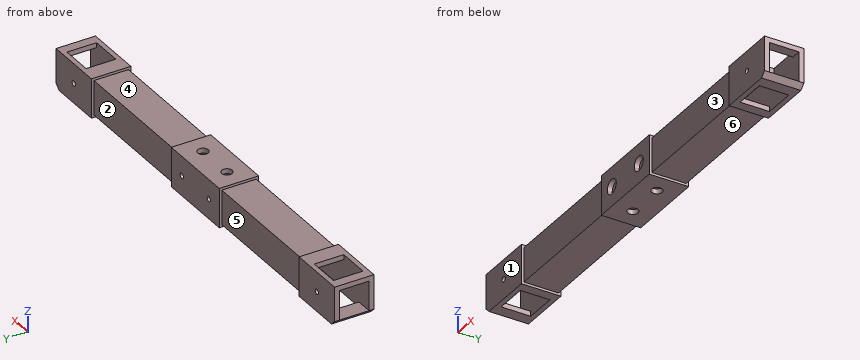
```python
from build123d import *

# Parameters (mm, degrees)
SKETCH1_W               = 50.8
SKETCH1_H               = 50.8
SKETCH1_W_2             = 38.1
SKETCH1_H_2             = 38.1
EXTRUDE1_DEPTH          = 355.6
F_1_2_CLEARANCE_HOLE1_D = 13.49248
EXTRUDE3_REACH          = 362.107
SKETCH6_W               = 40.64
SKETCH6_H               = 38.1
EXTRUDE4_REACH          = 362.107
SKETCH7_W               = 40.64
SKETCH7_H               = 38.1
SKETCH8_W               = 48.26
SKETCH8_H               = 50.8
EXTRUDE5_DEPTH          = 361.10715072
F_1_4_CLEARANCE_HOLE1_D = 6.7564
F_1_4_CLEARANCE_HOLE2_D = 6.7564
EXTRUDE6_DEPTH          = 361.10715072
EXTRUDE8_REACH          = 314.544
SKETCH17_R              = 9.525
SKETCH18_W              = 12.7
SKETCH18_H              = 50.8
EXTRUDE9_DEPTH          = 313.54387788
SKETCH19_W              = 168.91
SKETCH19_H              = 50.8
EXTRUDE10_DEPTH         = 3.175
SKETCH20_W              = 168.91
SKETCH20_H              = 44.45
EXTRUDE11_DEPTH         = 3.175
MIRROR5_COPY_1_SKETCH_W = 168.91
MIRROR5_COPY_1_SKETCH_H = 50.8
MIRROR5_COPY_1_DEPTH    = 3.175
MIRROR5_COPY_2_SKETCH_W = 168.91
MIRROR5_COPY_2_SKETCH_H = 44.45
MIRROR5_COPY_2_DEPTH    = 3.175


with BuildPart() as part:
    # Sketch1 → Extrude1 (new, symmetric)
    with BuildSketch(Plane(origin=(0, 0, 0), x_dir=(0, 0, -1), z_dir=(1, 0, 0))):
        Rectangle(SKETCH1_W, SKETCH1_H)
        Rectangle(SKETCH1_W_2, SKETCH1_H_2, mode=Mode.SUBTRACT)
    extrude(amount=EXTRUDE1_DEPTH, both=True)

    # 1/2 Clearance Hole1 (through all)
    with Locations(Plane.XY.offset(25.4)):
        with Locations((25.4, 0), (-25.4, 0)):
            Hole(F_1_2_CLEARANCE_HOLE1_D / 2)

    # Sketch6 → Extrude3 (cut, up to next)
    with BuildSketch(Plane.XY.offset(25.4), mode=Mode.PRIVATE) as extrude3_sk1:
        with Locations((-261.62, 0)):
            Rectangle(SKETCH6_W, SKETCH6_H)
    extrude3_tool1 = extrude(extrude3_sk1.sketch, amount=-EXTRUDE3_REACH, mode=Mode.PRIVATE) & part.part
    extrude3 = extrude3_tool1.solids().sort_by_distance((-261.62, 0, 25.4))[0]
    add(extrude3, mode=Mode.SUBTRACT)

    # Sketch7 → Extrude4 (cut, up to next)
    with BuildSketch(Plane(origin=(0, 0, -25.4), x_dir=(-1, 0, 0), z_dir=(0, 0, -1)), mode=Mode.PRIVATE) as extrude4_sk1:
        with Locations((252.73, 0)):
            Rectangle(SKETCH7_W, SKETCH7_H)
    extrude4_tool1 = extrude(extrude4_sk1.sketch, amount=-EXTRUDE4_REACH, mode=Mode.PRIVATE) & part.part
    extrude4 = extrude4_tool1.solids().sort_by_distance((-252.73, 0, -25.4))[0]
    add(extrude4, mode=Mode.SUBTRACT)

    # Sketch8 → Extrude5 (cut, through all)
    with BuildSketch(Plane.XY.offset(25.4)):
        with Locations((-331.47, 0)):
            Rectangle(SKETCH8_W, SKETCH8_H)
    extrude5 = extrude(amount=-EXTRUDE5_DEPTH, mode=Mode.SUBTRACT)

    # 1/4 Clearance Hole1 (through all)
    with Locations(Plane(origin=(0, 25.4, 0), x_dir=(-1, 0, 0), z_dir=(0, 1, 0))):
        with Locations((257.175, 0)):
            f_1_4_clearance_hole1 = Hole(F_1_4_CLEARANCE_HOLE1_D / 2)

    # 1/4 Clearance Hole2 (through all)
    with Locations(Plane(origin=(0, 25.4, 0), x_dir=(-1, 0, 0), z_dir=(0, 1, 0))):
        with Locations((28.575, 0)):
            f_1_4_clearance_hole2 = Hole(F_1_4_CLEARANCE_HOLE2_D / 2)

    # Sketch15 → Extrude6 (cut, through all)
    with BuildSketch(Plane(origin=(0, 25.4, 0), x_dir=(1, 0, 0), z_dir=(0, 1, 0))):
        Polygon((-307.34, 25.4), (-288.29, 25.4), (-307.34, 6.35), align=None)
    extrude6 = extrude(amount=-EXTRUDE6_DEPTH, mode=Mode.SUBTRACT)

    # Mirror1: Extrude3, Extrude4, Extrude5, 1/4 Clearance Hole1, 1/4 Clearance Hole2, Extrude6 across plane
    add(extrude3.mirror(Plane(origin=(0, 0, 0), x_dir=(0, 0, 1), z_dir=(1, 0, 0))), mode=Mode.SUBTRACT)
    add(extrude4.mirror(Plane(origin=(0, 0, 0), x_dir=(0, 0, 1), z_dir=(1, 0, 0))), mode=Mode.SUBTRACT)
    add(extrude5.mirror(Plane(origin=(0, 0, 0), x_dir=(0, 0, 1), z_dir=(1, 0, 0))), mode=Mode.SUBTRACT)
    add(f_1_4_clearance_hole1.mirror(Plane(origin=(0, 0, 0), x_dir=(0, 0, 1), z_dir=(1, 0, 0))), mode=Mode.SUBTRACT)
    add(f_1_4_clearance_hole2.mirror(Plane(origin=(0, 0, 0), x_dir=(0, 0, 1), z_dir=(1, 0, 0))), mode=Mode.SUBTRACT)
    add(extrude6.mirror(Plane(origin=(0, 0, 0), x_dir=(0, 0, 1), z_dir=(1, 0, 0))), mode=Mode.SUBTRACT)

    # Sketch17 → Extrude8 (cut, up to next)
    with BuildSketch(Plane.XZ.offset(25.4), mode=Mode.PRIVATE) as extrude8_sk1:
        with Locations(Location((-28.575, 0, 0), (0, 0, 270))):
            Circle(SKETCH17_R)
    extrude8_tool1 = extrude(extrude8_sk1.sketch, amount=-EXTRUDE8_REACH, mode=Mode.PRIVATE) & part.part
    # Sketch17 → Extrude8 (cut, up to next)
    with BuildSketch(Plane.XZ.offset(25.4), mode=Mode.PRIVATE) as extrude8_sk2:
        with Locations(Location((28.575, 0, 0), (0, 0, 270))):
            Circle(SKETCH17_R)
    extrude8_tool2 = extrude(extrude8_sk2.sketch, amount=-EXTRUDE8_REACH, mode=Mode.PRIVATE) & part.part
    add(extrude8_tool1.solids().sort_by_distance((-28.575, -25.4, 0))[0], mode=Mode.SUBTRACT)
    add(extrude8_tool2.solids().sort_by_distance((28.575, -25.4, 0))[0], mode=Mode.SUBTRACT)

    # Sketch18 → Extrude9 (cut, through all)
    with BuildSketch(Plane(origin=(0, 25.4, 0), x_dir=(1, 0, 0), z_dir=(0, 1, 0))):
        with Locations((-300.99, 0)):
            Rectangle(SKETCH18_W, SKETCH18_H)
    extrude9 = extrude(amount=-EXTRUDE9_DEPTH, mode=Mode.SUBTRACT)

    # Mirror2: Extrude9 across plane
    add(extrude9.mirror(Plane(origin=(0, 0, 0), x_dir=(0, 0, 1), z_dir=(1, 0, 0))), mode=Mode.SUBTRACT)

    # Sketch19 → Extrude10 (cut)
    with BuildSketch(Plane(origin=(0, 0, -25.4), x_dir=(-1, 0, 0), z_dir=(0, 0, -1))):
        with Locations((-135.255, 0)):
            Rectangle(SKETCH19_W, SKETCH19_H)
    extrude10 = extrude(amount=-EXTRUDE10_DEPTH, mode=Mode.SUBTRACT)

    # Mirror3: Extrude10 across plane
    add(extrude10.mirror(Plane.XY), mode=Mode.SUBTRACT)

    # Sketch20 → Extrude11 (cut)
    with BuildSketch(Plane.XZ.offset(25.4)):
        with Locations((135.255, 0)):
            Rectangle(SKETCH20_W, SKETCH20_H)
    extrude11 = extrude(amount=-EXTRUDE11_DEPTH, mode=Mode.SUBTRACT)

    # Mirror4: Extrude11 across plane
    add(extrude11.mirror(Plane.ZX), mode=Mode.SUBTRACT)

    # Mirror5: Extrude10, Extrude11 across plane
    add(extrude10.mirror(Plane(origin=(0, 0, 0), x_dir=(0, 0, 1), z_dir=(1, 0, 0))), mode=Mode.SUBTRACT)
    add(extrude11.mirror(Plane(origin=(0, 0, 0), x_dir=(0, 0, 1), z_dir=(1, 0, 0))), mode=Mode.SUBTRACT)

    # Mirror5 copy 1 sketch → Mirror5 copy 1 (cut)
    with BuildSketch(Plane.XY.offset(25.4)):
        with Locations((-135.255, 0)):
            Rectangle(MIRROR5_COPY_1_SKETCH_W, MIRROR5_COPY_1_SKETCH_H)
    extrude(amount=-MIRROR5_COPY_1_DEPTH, mode=Mode.SUBTRACT)

    # Mirror5 copy 2 sketch → Mirror5 copy 2 (cut)
    with BuildSketch(Plane(origin=(0, 25.4, 0), x_dir=(-1, 0, 0), z_dir=(0, 1, 0))):
        with Locations((135.255, 0)):
            Rectangle(MIRROR5_COPY_2_SKETCH_W, MIRROR5_COPY_2_SKETCH_H)
    extrude(amount=-MIRROR5_COPY_2_DEPTH, mode=Mode.SUBTRACT)


solid = part.part
```
Geometry: final body of the model. Coordinates: model frame, mm. Face numbers are marked on the shaded views. A direction names the side the tool comes from. Round coordinates to 2 decimals unless told otherwise and drop trailing zeros. Loops run counter-clockwise (first coordinate to the right, second up) from the corner with the lowest first, then second, coordinate; pieces in that order, holes last.
Item 1: Reachability of the marked faces 3, 4, 5 and 6 from +Z, -Z, +X, -X, +Y, -Y: full face, straight path, thin tool, end or side. Return the list, or none.
Checked values:
face 3: +Z, -Z, -Y
face 4: +Z, +Y, -Y
face 5: +Z, -Z, +Y
face 6: -Z, +Y, -Y
Item 2: Line query: L1, parallel to Z at x = -8, y = 18.5; L2, parallel to Y at x = -75.5, z = 5 (3 decimals). Output: solid intervals per line, ascending.
Checked values:
L1: z = -25.4 to -19.05, 19.05 to 25.4
L2: y = -22.225 to -19.05, 19.05 to 22.225
Item 3: Section B-B, the plane y = 0. State how many separate pieces and enclosed holes the cut face has, plus the area to 3 significant figures.
Checked values:
separate pieces: 10
enclosed holes: 0
area: 3,920 mm2
Item 4: Contact query for flat-ended pins moving along their axis: P1, Ø12, axis at x = 25.4, y = 0, coming from the +Z side; P2, Ø1.5, axis at x = -92, y = -9, coming from the +Z side (3 decimals); P3, Ø5, axis at y = -6.5, z = -22, coming from the +X side; P4, Ø2, axis at x = 142, z = 12.5, coming from the -Y side (3 decimals). Output: stop coordinate, or through.
Checked values:
P1: passes through
P2: stops at z = 22.225
P3: stops at x = 294.19
P4: stops at y = -22.225
Item 5: Mould query, pull axis X, two halves, no side actions, for the marked faces 1 and 2. Classes: released by +X, released by -X, zero draft, split by the parting line, or undercut.
Checked values:
face 1: zero draft
face 2: undercut
Item 6: Section C-C, the plane x = 137. Output: boundary loops of the cut face in (y, z) (3 decimals), plus the area to 3 significant figures.
Checked values:
outline: (-22.225, -22.225) - (22.225, -22.225) - (22.225, 22.225) - (-22.225, 22.225) - close; hole (-19.05, -19.05) - (19.05, -19.05) - (19.05, 19.05) - (-19.05, 19.05) - close
area: 524 mm2
Item 7: Section A-A, the plane x = -224.5. Output: boundary loops of the cut face in (y, z), plus the area to 3 significant figures.
Checked values:
outline: (-25.4, -25.4) - (25.4, -25.4) - (25.4, 25.4) - (-25.4, 25.4) - close; hole (-19.05, -19.05) - (19.05, -19.05) - (19.05, 19.05) - (-19.05, 19.05) - close
area: 1,130 mm2
